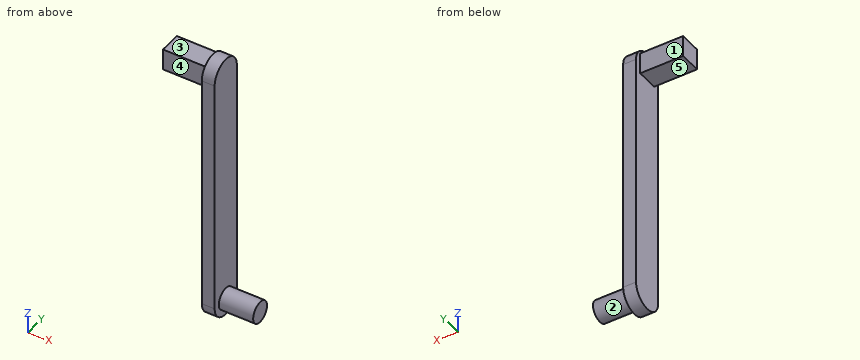
```python
from build123d import *

# Parameters (mm, degrees)
SKETCH1_R           = 3.81
BOSS_EXTRUDE1_DEPTH = 3.048
BOSS_EXTRUDE5_DEPTH = 3.81
SKETCH5_R           = 3.175
BOSS_EXTRUDE6_DEPTH = 10.16
SKETCH6_W           = 6.35
SKETCH6_H           = 6.35
BOSS_EXTRUDE7_DEPTH = 12.7


with BuildPart() as part:
    # Sketch1 → Boss-Extrude1 (new body)
    with BuildSketch(Plane(origin=(0, 0, 0), x_dir=(0, 0, -1), z_dir=(1, 0, 0))):
        Circle(SKETCH1_R)
    extrude(amount=BOSS_EXTRUDE1_DEPTH)

    # Sketch4 → Boss-Extrude5 (add)
    with BuildSketch(Plane(origin=(3.048, 0, 0), x_dir=(0, 0, -1), z_dir=(1, 0, 0))):
        with BuildLine():
            Line((0, 5.08), (71.12, 5.08))
            ThreePointArc((71.12, 5.08), (76.2, 0), (71.12, -5.08))
            Line((71.12, -5.08), (0, -5.08))
            ThreePointArc((0, -5.08), (-5.08, 0), (0, 5.08))
        make_face()
    extrude(amount=-BOSS_EXTRUDE5_DEPTH)

    # Sketch5 → Boss-Extrude6 (add)
    with BuildSketch(Plane(origin=(3.048, 0, 0), x_dir=(0, 0, -1), z_dir=(1, 0, 0))):
        with Locations((71.12, 0)):
            Circle(SKETCH5_R)
    extrude(amount=BOSS_EXTRUDE6_DEPTH)

    # Sketch6 → Boss-Extrude7 (add)
    with BuildSketch(Plane.ZY.offset(0.762)):
        Rectangle(SKETCH6_W, SKETCH6_H)
    extrude(amount=BOSS_EXTRUDE7_DEPTH)


solid = part.part
```
Can you work these out from the model? Positions are in its coordinate system, mm. Face numbers are marked on the shaded views. A direction names the side the tool comes from. Coordinates: 2 decimals unless noted, no trailing zeros. Order: outer loops, then holes, each group sorted by start corner. A loop starts at its lowest first (then second) coordinate and runs counter-clockwise, first axis right, second up.
1. I'm going to push flat-ended pins straight in: pin 1 (1.9 mm diameter, centred on x = -9.5, z = 1.5, fed in from -Y) (3 decimals); pin 2 (4 mm diameter, centred on x = -7, y = -3, fed in from +Z) (3 decimals); pin 3 (1.5 mm diameter, centred on x = 0.5, y = -1.5, fed in from -Z). Where does each tip first touch, or does it pass through?
2. If we section it at B-B (z = -59.5): Please give me the cut outline in (x, y).
3. I need wall thicknesses on line 1 (X direction, y = 3.5, z = -17); line 2 (Z direction, x = -10.75, y = -2.25) (3 decimals); line 3 (X direction, y = 0.25, z = -70). Which ranges of each line are inside material? Lowest first, please.
4. If we section it at C-C (x = -8): Please give me the cut outline in (y, z) (3 decimals).
5. For the marked faces 1, 2, 3, 4 and 5, which set-ups out of +Z, -Z, +X, -X, +Y, -Y let a thin tool reach every point of the face, with its end or its side?
6. If we section it at A-A (y = 0): Please give me the cut outline in (x, z) (3 decimals).
7. If we section it at D-D (x = 10.25): Please give me the cut outline in (y, z) (3 decimals), then the cut area to 3 significant figures.
Entries:
1. pin 1: stops at y = -3.175
1. pin 2: stops at z = 3.175
1. pin 3: stops at z = -76.14
2. outline: (-0.76, -5.08) - (3.05, -5.08) - (3.05, 5.08) - (-0.76, 5.08) - close
3. line 1: x = -0.76 to 3.05
3. line 2: z = -3.175 to 3.175
3. line 3: x = -0.76 to 13.21
4. outline: (-3.175, -3.175) - (3.175, -3.175) - (3.175, 3.175) - (-3.175, 3.175) - close
5. face 1: +Z, -Z, -X, +Y
5. face 2: +X
5. face 3: +Z, -X, +Y, -Y
5. face 4: +Z, -Z, -X, -Y
5. face 5: -Z, -X, +Y, -Y
6. outline: (-13.462, -3.175) - (-0.762, -3.175) - (-0.762, -76.2) - (3.048, -76.2) - (3.048, -74.295) - (13.208, -74.295) - (13.208, -67.945) - (3.048, -67.945) - (3.048, 5.08) - (-0.762, 5.08) - (-0.762, 3.175) - (-13.462, 3.175) - close
7. outline: circle Ø6.35 at (0, -71.12)
7. area: 31.7 mm2
